```python
from build123d import *

# Parameters (mm, degrees)
BOX002_W      = 3
BOX002_H      = 20
BOX002_DEPTH  = 5
BOX001_W      = 51
BOX001_H      = 20
BOX001_DEPTH  = 1
BOX_W         = 2
BOX_H         = 25
BOX_DEPTH     = 1
SKETCH_W      = 3
SKETCH_H      = 21
PAD_DEPTH     = 1
SKETCH001_W   = 5
SKETCH001_H   = 1.75
SKETCH001_H_2 = 1
PAD001_DEPTH  = 5
SKETCH002_W   = 3
SKETCH002_H   = 1
PAD002_DEPTH  = 2
SKETCH003_R   = 2.5
SKETCH003_R_2 = 1.3
PAD003_DEPTH  = 8.5
SKETCH004_W   = 16
SKETCH004_H   = 3.5
POCKET_DEPTH  = 1
CHAMFER_SIZE  = 0.5
SKETCH005_W   = 3
SKETCH005_H   = 1
PAD004_DEPTH  = 7
FILLET_R      = 1


with BuildPart() as obj1:
    # Box002 → Box002 (new body)
    with BuildSketch(Plane(origin=(-5, -25, -1), x_dir=(1, 0, 0), z_dir=(0, 0, 1))):
        with Locations((1.5, 10)):
            Rectangle(BOX002_W, BOX002_H)
    extrude(amount=BOX002_DEPTH)


with BuildPart() as wire_channel:
    # Box001 → Box001 (new body)
    with BuildSketch(Plane(origin=(-5, -25, -1), x_dir=(1, 0, 0), z_dir=(0, 0, 1))):
        with Locations((25.5, 10)):
            Rectangle(BOX001_W, BOX001_H)
    extrude(amount=BOX001_DEPTH)

    # Fusion: union obj1
    add(obj1.part)


with BuildPart() as obj2:
    # Box → Box (new body)
    with BuildSketch(Plane(origin=(43, -12.5, 1), x_dir=(1, 0, 0), z_dir=(0, 0, 1))):
        with Locations((1, 12.5)):
            Rectangle(BOX_W, BOX_H)
    extrude(amount=BOX_DEPTH)


with BuildPart() as cut001:
    # Sketch → Pad (new body)
    with BuildSketch(Plane.XY):
        Polygon((-45, 30), (45, 30), (45, -30), (-45, -30), (-45, -26.25), (-22, -26.25), (-22, -9.25), (-45, -9.25), (-45, -7.5), (-27, -7.5), (-27, 9.5), (-45, 9.5), (-45, 10.5), (-27, 10.5), (-27, 27.5), (-45, 27.5), align=None)
        Polygon((36.5, 21), (36.5, 28), (-16.5, 28), (-16.5, 21), (7, 21), (7, 19), (13, 19), (13, 21), align=None, mode=Mode.SUBTRACT)
        with Locations((5.5, 0)):
            Rectangle(SKETCH_W, SKETCH_H, mode=Mode.SUBTRACT)
        with Locations((11.5, 0)):
            Rectangle(SKETCH_W, SKETCH_H, mode=Mode.SUBTRACT)
        with Locations((17.5, 0)):
            Rectangle(SKETCH_W, SKETCH_H, mode=Mode.SUBTRACT)
        with Locations((23.5, 0)):
            Rectangle(SKETCH_W, SKETCH_H, mode=Mode.SUBTRACT)
    extrude(amount=PAD_DEPTH)

    # Sketch001 (on Face42 of Pad) → Pad001 (new body)
    with BuildSketch(Plane.XY.offset(1)):
        with Locations((-42.5, -8.375)):
            Rectangle(SKETCH001_W, SKETCH001_H)
        with Locations((-42.5, 10)):
            Rectangle(SKETCH001_W, SKETCH001_H_2)
        Polygon((-45, 30), (45, 30), (45, -30), (-45, -30), (-45, -26.25), (-40, -26.25), (-40, -29), (40, -29), (40, -27.5), (43.5, -27.5), (43.5, 27.5), (40, 27.5), (40, 29), (-40, 29), (-40, 27.5), (-45, 27.5), align=None)
    extrude(amount=PAD001_DEPTH)

    # Sketch002 (on Face56 of Pad001) → Pad002 (new body)
    with BuildSketch(Plane.XY.offset(6)):
        with Locations((41.5, 28)):
            Rectangle(SKETCH002_W, SKETCH002_H)
        with Locations((-41.5, 28)):
            Rectangle(SKETCH002_W, SKETCH002_H)
        with Locations((-41.5, -28)):
            Rectangle(SKETCH002_W, SKETCH002_H)
        with Locations((41.5, -28)):
            Rectangle(SKETCH002_W, SKETCH002_H)
    extrude(amount=PAD002_DEPTH)

    # Sketch003 (on Face47 of Pad002) → Pad003 (new body)
    with BuildSketch(Plane.XY.offset(1)):
        with Locations((-19, 24.5)):
            Circle(SKETCH003_R)
        with Locations((-19, 24.5)):
            Circle(SKETCH003_R_2, mode=Mode.SUBTRACT)
        with Locations((39, 24.5)):
            Circle(SKETCH003_R)
        with Locations((39, 24.5)):
            Circle(SKETCH003_R_2, mode=Mode.SUBTRACT)
        with Locations((-19, -24.5)):
            Circle(SKETCH003_R)
        with Locations((-19, -24.5)):
            Circle(SKETCH003_R_2, mode=Mode.SUBTRACT)
        with Locations((39, -24.5)):
            Circle(SKETCH003_R)
        with Locations((39, -24.5)):
            Circle(SKETCH003_R_2, mode=Mode.SUBTRACT)
    extrude(amount=PAD003_DEPTH)

    # Sketch004 (on Face45 of Pad003) → Pocket (cut)
    with BuildSketch(Plane.XZ.offset(30)):
        with BuildLine():
            ThreePointArc((-14.5, 6), (-11, 2.5), (-7.5, 6))
            Line((-14.5, 6), (-7.5, 6))
        make_face()
        with Locations((10.5, 4.25)):
            Rectangle(SKETCH004_W, SKETCH004_H)
    extrude(amount=-POCKET_DEPTH, mode=Mode.SUBTRACT)

    # Chamfer
    chamfer_edges = [cut001.edges().sort_by_distance(p)[0] for p in [
        (-20.3, 24.5, 9.5),
        (37.7, 24.5, 9.5),
        (37.7, -24.5, 9.5),
        (-20.3, -24.5, 9.5),
    ]]
    chamfer(chamfer_edges, length=CHAMFER_SIZE)

    # Sketch005 (on Face5 of Chamfer) → Pad004 (new body)
    with BuildSketch(Plane.XY.offset(1)):
        with Locations((42, -16.2)):
            Rectangle(SKETCH005_W, SKETCH005_H)
        with Locations((42, -19.5)):
            Rectangle(SKETCH005_W, SKETCH005_H)
    extrude(amount=PAD004_DEPTH)

    # Cut: cut obj2
    add(obj2.part, mode=Mode.SUBTRACT)

    # Fillet
    fillet_edges = [cut001.edges().sort_by_distance(p)[0] for p in [
        (43.5, 0, 2),
    ]]
    fillet(fillet_edges, radius=FILLET_R)

    # Cut001: cut wire channel
    add(wire_channel.part, mode=Mode.SUBTRACT)


solid = cut001.part
```
For this review, take the finished solid that the model builds, in its own axes (mm). A direction names the side the tool comes from. Round coordinates to 2 decimals unless told otherwise and drop trailing zeros. Write each loop counter-clockwise with the first axis right and the second up, starting at its lowest first coordinate (ties: lowest second). Pieces come first, ordered by that corner, then holes. Notation, with made-up numbers: M 48,33.25 L 67,33.25 A37 cw 67,70.25 Z; hole C 56.25,-8 d3. An arc over 180 degrees is marked long. One line per item, written item: value. Start each with the question number.
(1) We need section C-C (x = -11). Give the boundary of the cut face in (y, z).
(2) Wall thickness on line 1 (Y direction, x = -19, z = 3.25); line 2 (Y direction, x = -0.5, z = 4.5); line 3 (X direction, y = -8.5, z = 5): over which ranges is each line inside the solid? List them lowest first.
(3) Insertion check: pin 1 (4 mm diameter, centred on y = -5, z = 1.5, fed in from -X); pin 2 (0.5 mm diameter, centred on y = 28, z = 7.5, fed in from -X); pin 3 (0.8 mm diameter, centred on y = 28, z = 7, fed in from +X); pin 4 (4 mm diameter, centred on x = -1, z = 7.5, fed in from +Y). Each pin has a flat end and moves straight along its axis. Give the tip position at first contact, or say it passes through.
(4) We need section D-D (y = 3). Give the boundary of the cut face in (x, z).
(5) We need section A-A (x = -32). Give the boundary of the cut face in (y, z), and give its area (3 significant figures).
(6) We need section B-B (y = 11.5). Give the boundary of the cut face in (x, z).
(7) The part is to be moulded in two halves that separate along Y. For faces 1 (the flat face through (37, -24, 9.5)), 2 (the flat face through (-42, -28.5, 7)), 3 (the cylindrical face through (-21, -23, 5)), say which applies: released by +Y, released by -Y, zero draft, split by the parting line, or undercut.
(8) Machinability: for faces 4 (the flat face through (-38.8, -26.25, 0.3)), 5 (the flat face through (-19, 25, 1)), 6 (the flat face through (43.5, -18, 3)), which of the approach directions +Z, -Z, +X, -X, +Y, -Y give a long, thin tool a straight path to every point of the face, cutting with its end or side? Answer none if there is none.
Result:
1. outline: M -30,0 L 21,0 L 21,1 L -29,1 L -29,2.5 L -30,2.5 Z; M 28,0 L 30,0 L 30,6 L 29,6 L 29,1 L 28,1 Z
2. line 1: -30 to -29, -27 to -25.8, -23.2 to -22, 22 to 23.2, 25.8 to 27, 29 to 30
2. line 2: -30 to -29, 29 to 30
2. line 3: -45 to -40, 43.5 to 45
3. pin 1: x = -27
3. pin 2: x = -43
3. pin 3: x = 43
3. pin 4: y = 30
4. outline: M -27,0 L 4,0 L 4,1 L -27,1 Z; M 7,0 L 10,0 L 10,1 L 7,1 Z; M 13,0 L 16,0 L 16,1 L 13,1 Z; M 19,0 L 22,0 L 22,1 L 19,1 Z; M 25,0 L 45,0 L 45,1 L 25,1 Z; M 43.5,3 A1 ccw 44.5,2 L 45,2 L 45,6 L 43.5,6 Z
5. outline: M -30,0 L -26.25,0 L -26.25,1 L -29,1 L -29,6 L -30,6 Z; M -9.25,0 L -7.5,0 L -7.5,1 L -9.25,1 Z; M 9.5,0 L 10.5,0 L 10.5,1 L 9.5,1 Z; M 27.5,0 L 30,0 L 30,6 L 29,6 L 29,1 L 27.5,1 Z
5. area: 19.0 mm²
6. outline: M -27,0 L 45,0 L 45,1 L -27,1 Z; M 43.5,3 A1 ccw 44.5,2 L 45,2 L 45,6 L 43.5,6 Z
7. face 1: zero draft
7. face 2: released by -Y
7. face 3: undercut
8. face 4: +Z, -Z, -X
8. face 5: +Z
8. face 6: +Z, -X
